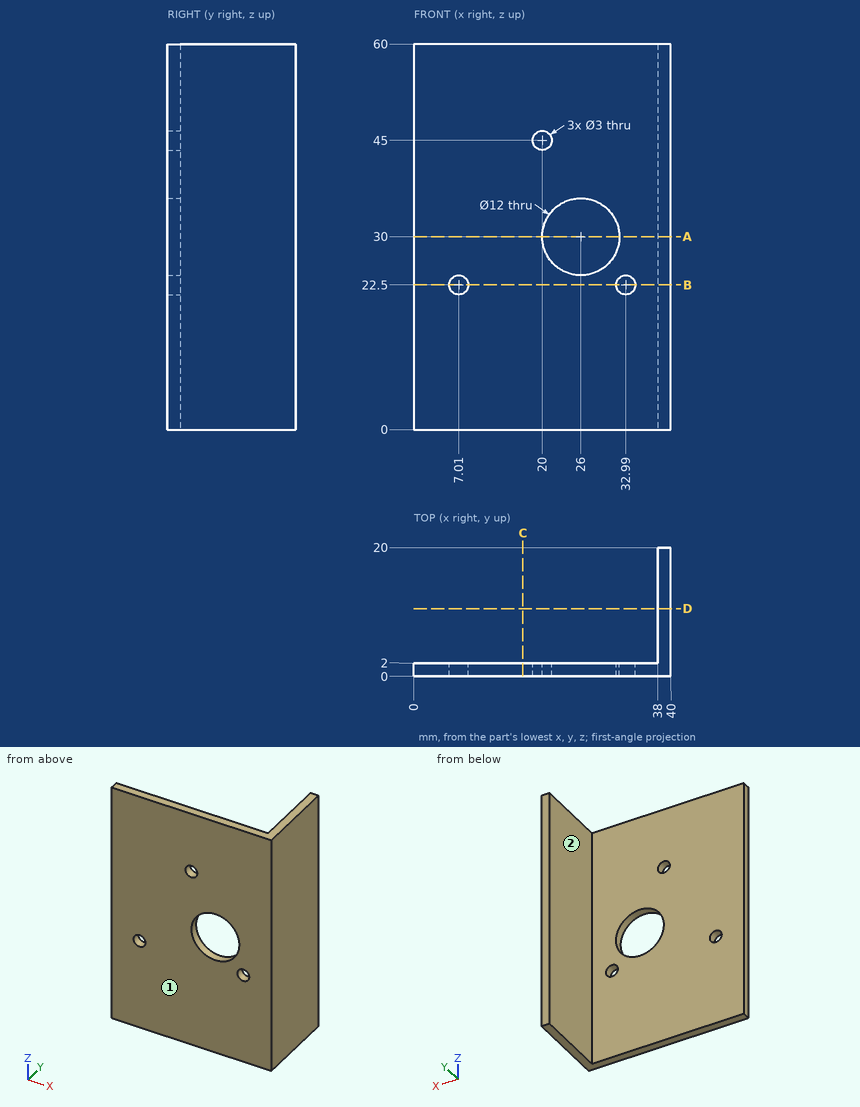
Here's the drawing with two shaded views (mm, measured from the low corner). I have some questions. A direction names the side the tool comes from. Give positions to 0.01 mm unless a question says otherwise; leave off trailing zeros. Write each loop counter-clockwise with the first axis right and the second up, starting at its lowest first coordinate (ties: lowest second). Pieces come first, ordered by that corner, then holes. Notation, with made-up numbers: (-18.75, -22) -> (-13.75, -22) arc R35 cw to (-13.75, 17) -> close; hole circle Ø4 at (-9.5, 56.25). An arc over 180 degrees is marked (long way). Answer as a JSON object with one key per item and string values. Group by question number.
Item 1: Suppose I cut it at C-C (x = 17). Please give me the cut outline in (y, z).
Item 2: Suppose I cut it at A-A (z = 30). Please give me the cut outline in (x, y).
Item 3: Please list where these lines run through material, in increasing order: line 1 (Z direction, x = 26, y = 0.9); line 2 (X direction, y = 1.45, z = 45); line 3 (Y direction, x = 18, z = 36.5). Write a range as [from, to].
Item 4: For the marked faces 1 and 2, which set-ups out of +Z, -Z, +X, -X, +Y, -Y let a thin tool reach every point of the face, with its end or its side?
Item 5: I'm going to push flat-ended pins straight in: P1, Ø5, axis at y = 9, z = 41.5, coming from the -X side; P2, Ø4, axis at x = 35.5, z = 15, coming from the +Y side. Where does each tip first touch, or does it pass through?
Item 6: Suppose I cut it at B-B (z = 22.5). Please give me the cut outline in (x, y), plus the area to 3 significant figures.
Item 7: Suppose I cut it at D-D (y = 10.5). Please give me the cut outline in (x, z), plus the area to 3 significant figures.
Findings:
{
 "1": {"outline": "(0, 0) -> (2, 0) -> (2, 60) -> (0, 60) -> close"},
 "2": {"outline": "(0, 0) -> (20, 0) -> (20, 2) -> (0, 2) -> close; (32, 0) -> (40, 0) -> (40, 20) -> (38, 20) -> (38, 2) -> (32, 2) -> close"},
 "3": {"line 1": "z = [0, 24], [36, 60]", "line 2": "x = [0, 18.5], [21.5, 40]", "line 3": "y = [0, 2]"},
 "4": {"face 1": "+Z, -Z, +X, -X, -Y", "face 2": "+Z, -Z, -X, +Y"},
 "5": {"P1": "stops at x = 38", "P2": "stops at y = 2"},
 "6": {"outline": "(0, 0) -> (5.51, 0) -> (5.51, 2) -> (0, 2) -> close; (8.51, 0) -> (31.49, 0) -> (31.49, 2) -> (8.51, 2) -> close; (34.49, 0) -> (40, 0) -> (40, 20) -> (38, 20) -> (38, 2) -> (34.49, 2) -> close", "area": "104 mm²"},
 "7": {"outline": "(38, 0) -> (40, 0) -> (40, 60) -> (38, 60) -> close", "area": "120 mm²"}
}
